Model file for the job. Use its own axes, mm. A direction names the side the tool comes from. Give positions to 0.01 mm unless a question says otherwise; leave off trailing zeros. Loops run counter-clockwise (first coordinate to the right, second up) from the corner with the lowest first, then second, coordinate; pieces in that order, holes last. Notation, with made-up numbers: M 89.25,46 L 102.25,46 A17 ccw 102.25,52 Z; hole C -40,-37.5 d1. An arc over 180 degrees is marked long. Answer in a Markdown table with one row per item.
```python
from build123d import *

# Parameters (mm, degrees)
PAD_DEPTH       = 3
SKETCH001_R     = 7
POCKET_DEPTH    = 3.001
SKETCH002_W     = 30
SKETCH002_H     = 19.5
PAD001_DEPTH    = 3
SKETCH003_W     = 30
SKETCH003_H     = 19.5
PAD002_DEPTH    = 3
SKETCH004_W     = 40
SKETCH004_H     = 19.5
PAD003_DEPTH    = 3
SKETCH005_W     = 40
SKETCH005_H     = 19.5
PAD004_DEPTH    = 3
SKETCH006_W     = 23.5
SKETCH006_H     = 40
SKETCH006_W_2   = 30
SKETCH006_H_2   = 12.5
PAD005_DEPTH    = 5
SKETCH007_R     = 1.65
POCKET001_DEPTH = 5.001
POCKET002_DEPTH = 2
FILLET_R        = 1
FILLET001_R     = 1
FILLET002_R     = 1
FILLET003_R     = 1
FILLET004_R     = 1
FILLET005_R     = 1
FILLET006_R     = 1
FILLET007_R     = 1


with BuildPart() as part:
    # Sketch → Pad (new body)
    with BuildSketch(Plane.XY):
        Polygon((-51.5, -20), (-51.5, 20), (-15, 20), (-15, 37.5), (15, 37.5), (15, 20), (51.5, 20), (51.5, -20), (15, -20), (15, -37.5), (-15, -37.5), (-15, -20), align=None)
    extrude(amount=PAD_DEPTH)

    # Sketch001 (on Face14 of Pad) → Pocket (cut, through all)
    with BuildSketch(Plane.XY.offset(3)):
        with Locations((-40, 0)):
            Circle(SKETCH001_R)
        with Locations((-20, 0)):
            Circle(SKETCH001_R)
        Circle(SKETCH001_R)
        with Locations((20, 0)):
            Circle(SKETCH001_R)
        with Locations((40, 0)):
            Circle(SKETCH001_R)
        with Locations((0, -20)):
            Circle(SKETCH001_R)
        with Locations((0, 20)):
            Circle(SKETCH001_R)
    extrude(amount=-POCKET_DEPTH, mode=Mode.SUBTRACT)

    # Sketch002 (on Face8 of Pocket) → Pad001 (join)
    with BuildSketch(Plane.XZ.offset(37.5)):
        with Locations((0, 9.75)):
            Rectangle(SKETCH002_W, SKETCH002_H)
    extrude(amount=PAD001_DEPTH)

    # Sketch003 (on Face9 of Pad001) → Pad002 (join)
    with BuildSketch(Plane(origin=(0, 37.5, 0), x_dir=(-1, 0, 0), z_dir=(0, 1, 0))):
        with Locations((0, 9.75)):
            Rectangle(SKETCH003_W, SKETCH003_H)
    extrude(amount=PAD002_DEPTH)

    # Sketch004 (on Face1 of Pad002) → Pad003 (join)
    with BuildSketch(Plane(origin=(-51.5, 0, 0), x_dir=(0, -1, 0), z_dir=(-1, 0, 0))):
        with Locations((0, 9.75)):
            Rectangle(SKETCH004_W, SKETCH004_H)
    extrude(amount=PAD003_DEPTH)

    # Sketch005 (on Face19 of Pad003) → Pad004 (join)
    with BuildSketch(Plane.YZ.offset(51.5)):
        with Locations((0, 9.75)):
            Rectangle(SKETCH005_W, SKETCH005_H)
    extrude(amount=PAD004_DEPTH)

    # Sketch006 (on Face8 of Pad004) → Pad005 (join)
    with BuildSketch(Plane.XY.offset(19.5)):
        with Locations((-63.25, 0)):
            Rectangle(SKETCH006_W, SKETCH006_H)
        with Locations((63.25, 0)):
            Rectangle(SKETCH006_W, SKETCH006_H)
        with Locations((0, 43.75)):
            Rectangle(SKETCH006_W_2, SKETCH006_H_2)
        with Locations((0, -43.75)):
            Rectangle(SKETCH006_W_2, SKETCH006_H_2)
    extrude(amount=-PAD005_DEPTH)

    # Sketch007 (on Face60 of Pad005) → Pocket001 (cut, through all)
    with BuildSketch(Plane(origin=(0, 0, 14.5), x_dir=(1, 0, 0), z_dir=(0, 0, -1))):
        with Locations((-69, 10.5)):
            Circle(SKETCH007_R)
        with Locations((69, 10.5)):
            Circle(SKETCH007_R)
        with Locations((0, 44.5)):
            Circle(SKETCH007_R)
        with Locations((0, -44.5)):
            Circle(SKETCH007_R)
        with Locations((-69, -10.5)):
            Circle(SKETCH007_R)
        with Locations((69, -10.5)):
            Circle(SKETCH007_R)
    extrude(amount=-POCKET001_DEPTH, mode=Mode.SUBTRACT)

    # Sketch008 (on Face36 of Pocket001) → Pocket002 (cut)
    with BuildSketch(Plane(origin=(0, 0, 14.5), x_dir=(1, 0, 0), z_dir=(0, 0, -1))):
        Polygon((-65.95, 8.739082), (-65.95, 12.260918), (-69, 14.021837), (-72.05, 12.260918), (-72.05, 8.739082), (-69, 6.978163), align=None)
        Polygon((-65.95, -12.260918), (-65.95, -8.739082), (-69, -6.978163), (-72.05, -8.739082), (-72.05, -12.260918), (-69, -14.021837), align=None)
        Polygon((72.05, 8.739082), (72.05, 12.260918), (69, 14.021837), (65.95, 12.260918), (65.95, 8.739082), (69, 6.978163), align=None)
        Polygon((72.05, -12.260918), (72.05, -8.739082), (69, -6.978163), (65.95, -8.739082), (65.95, -12.260918), (69, -14.021837), align=None)
        Polygon((1.760918, 41.45), (3.521837, 44.5), (1.760918, 47.55), (-1.760918, 47.55), (-3.521837, 44.5), (-1.760918, 41.45), align=None)
        Polygon((1.760918, -47.55), (3.521837, -44.5), (1.760918, -41.45), (-1.760918, -41.45), (-3.521837, -44.5), (-1.760918, -47.55), align=None)
    extrude(amount=-POCKET002_DEPTH, mode=Mode.SUBTRACT)

    # Fillet
    fillet_edges = [part.edges().sort_by_distance(p)[0] for p in [
        (-75, 0, 14.5),
    ]]
    fillet(fillet_edges, radius=FILLET_R)

    # Fillet001
    fillet001_edges = [part.edges().sort_by_distance(p)[0] for p in [
        (0, 50, 14.5),
    ]]
    fillet(fillet001_edges, radius=FILLET001_R)

    # Fillet002
    fillet002_edges = [part.edges().sort_by_distance(p)[0] for p in [
        (0, -50, 14.5),
    ]]
    fillet(fillet002_edges, radius=FILLET002_R)

    # Fillet003
    fillet003_edges = [part.edges().sort_by_distance(p)[0] for p in [
        (75, 0, 14.5),
    ]]
    fillet(fillet003_edges, radius=FILLET003_R)

    # Fillet004
    fillet004_edges = [part.edges().sort_by_distance(p)[0] for p in [
        (54.5, 0, 0),
    ]]
    fillet(fillet004_edges, radius=FILLET004_R)

    # Fillet005
    fillet005_edges = [part.edges().sort_by_distance(p)[0] for p in [
        (0, 40.5, 0),
    ]]
    fillet(fillet005_edges, radius=FILLET005_R)

    # Fillet006
    fillet006_edges = [part.edges().sort_by_distance(p)[0] for p in [
        (-54.5, 0, 0),
    ]]
    fillet(fillet006_edges, radius=FILLET006_R)

    # Fillet007
    fillet007_edges = [part.edges().sort_by_distance(p)[0] for p in [
        (0, -40.5, 0),
    ]]
    fillet(fillet007_edges, radius=FILLET007_R)


solid = part.part
```
Q1. Drop flat-ended pins along their axis: pin 1 (8.5 mm diameter, centred on x = -40, y = 0, fed in from -Z); pin 2 (10 mm diameter, centred on x = -57, z = 13.5, fed in from +Y); pin 3 (10 mm diameter, centred on y = -6, z = 3, fed in from +X); pin 4 (10 mm diameter, centred on x = -44.5, z = 5.5, fed in from -Y). Give the stop position or say it passes through.
Reported:
| item | result |
|---|---|
| pin 1 | through |
| pin 2 | y = 20 |
| pin 3 | x = 54.5 |
| pin 4 | y = -20 |
Q2. 3-axis set-ups, long thin cutter, end or side, ignore diameter. For faces 5 (the face through (-52, 20, 10)), 6 (the face through (-52, -20, 10)), 7 (the face through (0, -37.5, 11)): which of +Z, -Z, +X, -X, +Y, -Y reach the whole face in a straight line?
Reported:
| item | result |
|---|---|
| face 5 | +Z, -Z, -X, +Y |
| face 6 | +Z, -Z, -X, -Y |
| face 7 | +Z, +X, -X |
Q3. Saw through at D-D (y = -22). Give the cut face in (x, z), and give its area (3 significant figures).
Reported:
| item | result |
|---|---|
| outline | M -15,0 L -6.71,0 L -6.71,3 L -15,3 Z; M 6.71,0 L 15,0 L 15,3 L 6.71,3 Z |
| area | 49.8 mm² |
Q4. Mould opens along X. For faces 1 (the face through (0, 37.5, 11)), 2 (the face through (51.5, 0, 11)), 3 (the face through (-15, 38, 8)), 4 (the face through (67.35, -10.57, 17.98)) say: released by +X, released by -X, zero draft, split by the parting line, or undercut.
Reported:
| item | result |
|---|---|
| face 1 | zero draft |
| face 2 | undercut |
| face 3 | released by -X |
| face 4 | undercut |
Q5. Saw through at B-B (y = -10.5). Give the number of separate pieces and of enclosed holes in the cut face, and give its area (3 significant figures).
Reported:
| item | result |
|---|---|
| separate pieces | 3 |
| enclosed holes | 0 |
| area | 586 mm² |
Q6. Saw through at A-A (x = 20). Give the cut face in (y, z), and give its area (3 significant figures).
Reported:
| item | result |
|---|---|
| outline | M -20,0 L -7,0 L -7,3 L -20,3 Z; M 7,0 L 20,0 L 20,3 L 7,3 Z |
| area | 78.0 mm² |
Q7. Probe probe 1 along Y at (x, z) = (0, 0.95); probe 2 along X at (y, z) = (-1, 7.5); probe 3 along X at (y, z) = (-44.5, 18.65). List the from-to ranges inside material, lowest first.
Reported:
| item | result |
|---|---|
| probe 1 | -40.5 to -27, -13 to -7, 7 to 13, 27 to 40.5 |
| probe 2 | -54.5 to -51.5, 51.5 to 54.5 |
| probe 3 | -15 to -1.65, 1.65 to 15 |
Q8. Saw through at C-C (z = 6.25). Give the cut face in (x, y).
Reported:
| item | result |
|---|---|
| outline | M -54.5,-20 L -51.5,-20 L -51.5,20 L -54.5,20 Z; M -15,-40.5 L 15,-40.5 L 15,-37.5 L -15,-37.5 Z; M -15,37.5 L 15,37.5 L 15,40.5 L -15,40.5 Z; M 51.5,-20 L 54.5,-20 L 54.5,20 L 51.5,20 Z |
